For this review, take the finished solid that the model builds, in its own axes (mm). A direction names the side the tool comes from. Coordinates: 2 decimals unless noted, no trailing zeros. Loops run counter-clockwise (first coordinate to the right, second up) from the corner with the lowest first, then second, coordinate; pieces in that order, holes last. Notation, with made-up numbers: (67, 46.25) - (109, 46.25) arc R22 cw to (109, 65.25) - close; hole circle Ø6 at (-14.5, 89.25). An arc over 180 degrees is marked (long way). Use one line per item in the form item = value. Start each with the question number.
1. To check wall thickness, follow probe 1 along X at (y, z) = (14.75, 5.5); probe 2 along X at (y, z) = (8.5, 5); probe 3 along Y at (x, z) = (9.5, 4.25). State the ranges of each line that lie inside material, in increasing order.
2. Add section D-D on y = 10.25. Give the boundary of the cut face in (x, z), and give its area (3 significant figures).
3. Add section C-C on x = 14.5. Give the boundary of the cut face in (y, z).
4. Add section A-A on y = 15.75. Give the boundary of the cut face in (x, z), and give its area (3 significant figures).
5. Machinability: for faces 4 (the face through (15, 17, 4)), 5 (the face through (15, 11, 0.814)), 6 (the face through (13.89, 8, 6)), which of the approach directions +Z, -Z, +X, -X, +Y, -Y give a long, thin tool a straight path to every point of the face, cutting with its end or side? Answer none if there is none.
6. For pin 1 Ø4 at (y, z) = (11.5, 3) entering from +X; pin 2 Ø0.6 at (x, z) = (14.5, 4) entering from +Y, all flat-tipped, find the tip position at first contact; note any pin that passes through.
7. Add section B-B on z = 2. Give the boundary of the cut face in (x, y), and give its area (3 significant figures).
8. Draft analysis for pull direction Y (two halves, no side actions). For faces 1 (the face through (8, 0, 4)), 2 (the face through (6.858, 8, 4)), 3 (the face through (7.89, 9.76, 3.18)), state which applies: +Y half, -Y half, draft (parallel to the pull), parting line (faces both ways), or undercut.
```python
from build123d import *

# Parameters (mm, degrees)
EXTRUSION1_DEPTH   = 8.128
SKETCH2_R          = 1.4605
CUT_EXTRUDE2_DEPTH = 10
CUT_EXTRUDE3_REACH = 27.212


with BuildPart() as part:
    # Sketch1 → Extrusion1 (new body)
    with BuildSketch(Plane.XY):
        Polygon((0, 17.78), (2.032, 17.78), (2.032, 2.286), (6.858, 2.286), (6.858, 17.78), (8.89, 17.78), (8.89, 0), (0, 0), (0, 2.154296207), align=None)
        Polygon((8.89, 2.286), (8.89, 0), (15.24, 0), (15.92, 0), (15.92, 17), (13.89, 17), (13.89, 2.286), align=None)
    extrude(amount=EXTRUSION1_DEPTH)

    # Sketch2 → Cut-Extrude2 (cut)
    with BuildSketch(Plane(origin=(8.89, 0, 0), x_dir=(0, 0, -1), z_dir=(1, 0, 0))):
        with Locations(Location((-4.064, 10.922, 0), (0, 0, 90))):
            Circle(SKETCH2_R)
    extrude(amount=-CUT_EXTRUDE2_DEPTH, mode=Mode.SUBTRACT)

    # Sketch4 → Cut-Extrude3 (cut, up to next)
    with BuildSketch(Plane(origin=(15.92, 0, 0), x_dir=(0, 0, -1), z_dir=(1, 0, 0)), mode=Mode.PRIVATE) as cut_extrude3_sk1:
        Polygon((-4.064, 14.67477675), (-7.314, 12.798388375), (-7.314, 9.045611625), (-4.064, 7.16922325), (-0.814, 9.045611625), (-0.814, 12.798388375), align=None)
    cut_extrude3_tool1 = extrude(cut_extrude3_sk1.sketch, amount=-CUT_EXTRUDE3_REACH, mode=Mode.PRIVATE) & part.part
    add(cut_extrude3_tool1.solids().sort_by_distance((15.92, 10.922, 4.064))[0], mode=Mode.SUBTRACT)


solid = part.part
```
Conclusion:
q1.probe_1 = 0 to 2.03, 6.86 to 8.89, 13.89 to 15.92
q1.probe_2 = 0 to 2.03, 6.86 to 8.89
q1.probe_3 = 0 to 2.29
q2.outline = (0, 0) - (2.03, 0) - (2.03, 2.77) - (0, 2.77) - close; (0, 5.36) - (2.03, 5.36) - (2.03, 8.13) - (0, 8.13) - close; (6.86, 0) - (8.89, 0) - (8.89, 2.77) - (6.86, 2.77) - close; (6.86, 5.36) - (8.89, 5.36) - (8.89, 8.13) - (6.86, 8.13) - close; (13.89, 0) - (15.92, 0) - (15.92, 0.81) - (13.89, 0.81) - close; (13.89, 7.31) - (15.92, 7.31) - (15.92, 8.13) - (13.89, 8.13) - close
q2.area = 25.8 mm^2
q3.outline = (0, 0) - (17, 0) - (17, 8.13) - (0, 8.13) - close; hole (7.17, 4.06) - (9.05, 0.81) - (12.8, 0.81) - (14.67, 4.06) - (12.8, 7.31) - (9.05, 7.31) - close
q4.outline = (0, 0) - (2.03, 0) - (2.03, 8.13) - (0, 8.13) - close; (6.86, 0) - (8.89, 0) - (8.89, 8.13) - (6.86, 8.13) - close; (13.89, 0) - (15.92, 0) - (15.92, 8.13) - (13.89, 8.13) - close
q4.area = 49.5 mm^2
q5.face_4 = +Z, -Z, +X, +Y
q5.face_5 = +X
q5.face_6 = +Z, -Z, +Y
q6.pin_1 = 8.89
q6.pin_2 = 17
q7.outline = (0, 0) - (15.92, 0) - (15.92, 8.36) - (13.89, 8.36) - (13.89, 2.29) - (8.89, 2.29) - (8.89, 17.78) - (6.86, 17.78) - (6.86, 2.29) - (2.03, 2.29) - (2.03, 17.78) - (0, 17.78) - close; (13.89, 13.48) - (15.92, 13.48) - (15.92, 17) - (13.89, 17) - close
q7.area = 119 mm^2
q8.face_1 = -Y half
q8.face_2 = draft
q8.face_3 = undercut
